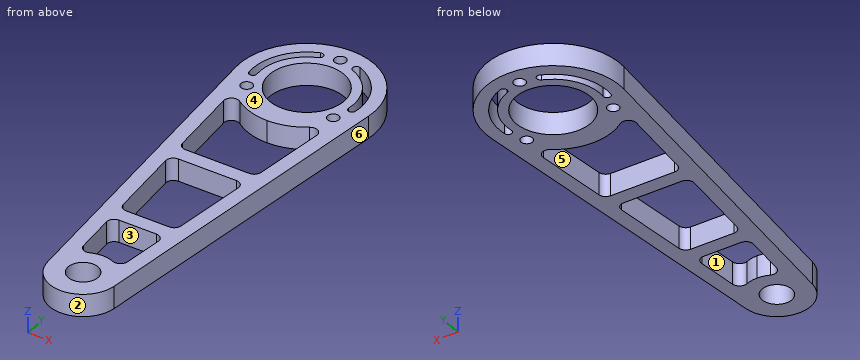
```python
from build123d import *

# Parameters (mm, degrees)
SKETCH_1_R          = 4
SKETCH_1_R_2        = 1.55
SKETCH_1_R_3        = 10
EXTRUDE_1_DEPTH     = 6
CUT_EXTRUDE_1_DEPTH = 6
EXTRUDE_2_DEPTH     = 6
FILLET_1_R          = 2
CUT_EXTRUDE_2_DEPTH = 10


with BuildPart() as part:
    # 草图1 → 凸台-拉伸1 (new body)
    with BuildSketch(Plane.XY):
        with BuildLine():
            ThreePointArc((17.909773868, -1.8), (0, 18), (-17.909773868, -1.8))
            Line((-17.909773868, -1.8), (-8.954886934, -90.9))
            ThreePointArc((-8.954886934, -90.9), (0, -99), (8.954886934, -90.9))
            Line((8.954886934, -90.9), (17.909773868, -1.8))
        make_face()
        with Locations((0, -90)):
            Circle(SKETCH_1_R, mode=Mode.SUBTRACT)
        with Locations((-11.691342951, -6.75)):
            Circle(SKETCH_1_R_2, mode=Mode.SUBTRACT)
        with Locations((11.691342951, -6.75)):
            Circle(SKETCH_1_R_2, mode=Mode.SUBTRACT)
        Circle(SKETCH_1_R_3, mode=Mode.SUBTRACT)
        with Locations((0, 13.5)):
            Circle(SKETCH_1_R_2, mode=Mode.SUBTRACT)
    extrude(amount=EXTRUDE_1_DEPTH)

    # 草图2 → 切除-拉伸1 (cut)
    with BuildSketch(Plane.XY.offset(6)):
        with BuildLine():
            ThreePointArc((13.15522745, -9.107139547), (7.425825451, -14.172406866), (0, -16))
            Line((0, -16), (0, -82))
            ThreePointArc((0, -82), (3.024106775, -82.593598835), (5.599436985, -84.286305447))
            Line((5.599436985, -84.286305447), (13.15522745, -9.107139547))
        make_face()
        with BuildLine():
            ThreePointArc((0, -16), (-7.425825451, -14.172406866), (-13.15522745, -9.107139547))
            Line((-13.15522745, -9.107139547), (-5.599436985, -84.286305447))
            ThreePointArc((-5.599436985, -84.286305447), (-3.024106775, -82.593598835), (0, -82))
            Line((0, -82), (0, -16))
        make_face()
    extrude(amount=-CUT_EXTRUDE_1_DEPTH, mode=Mode.SUBTRACT)

    # 草图3 → 凸台-拉伸2 (add)
    with BuildSketch(Plane.XY.offset(6)):
        Polygon((10.251385716, -38), (-10.251385716, -38), (-10.050378153, -40), (10.050378153, -40), align=None)
        Polygon((-10.452393279, -36), (-10.251385716, -38), (10.251385716, -38), (10.452393279, -36), align=None)
        Polygon((7.437279833, -66), (-7.437279833, -66), (-7.23627227, -68), (7.23627227, -68), align=None)
        Polygon((7.638287396, -64), (-7.638287396, -64), (-7.437279833, -66), (7.437279833, -66), align=None)
    extrude(amount=-EXTRUDE_2_DEPTH)

    # 圆角1
    fillet_1_edges = [part.edges().sort_by_distance(p)[0] for p in [
        (-13.15522745, -9.107139547, 3),
        (13.15522745, -9.107139547, 3),
        (5.599436985, -84.286305447, 3),
        (-5.599436985, -84.286305447, 3),
        (-10.050378153, -40, 3),
        (-10.452393279, -36, 3),
        (10.452393279, -36, 3),
        (10.050378153, -40, 3),
        (-7.23627227, -68, 3),
        (-7.638287396, -64, 3),
        (7.638287396, -64, 3),
        (7.23627227, -68, 3),
    ]]
    fillet(fillet_1_edges, radius=FILLET_1_R)

    # 草图4 → 切除-拉伸2 (cut)
    with BuildSketch(Plane.XY.offset(6)):
        with BuildLine():
            ThreePointArc((-4.62962963, 11.611052041), (-4.071115837, 12.910306574), (-5.37037037, 13.468820367))
            ThreePointArc((-5.37037037, 13.468820367), (-12.505593382, 7.338946393), (-14.377656014, -1.87962963))
            ThreePointArc((-14.377656014, -1.87962963), (-13.256463901, -2.741562484), (-12.394531047, -1.62037037))
            ThreePointArc((-12.394531047, -1.62037037), (-10.78068395, 6.326677925), (-4.62962963, 11.611052041))
        make_face()
        with BuildLine():
            ThreePointArc((5.37037037, 13.468820367), (12.505593382, 7.338946393), (14.377656014, -1.87962963))
            ThreePointArc((14.377656014, -1.87962963), (13.256463901, -2.741562484), (12.394531047, -1.62037037))
            ThreePointArc((12.394531047, -1.62037037), (10.78068395, 6.326677925), (4.62962963, 11.611052041))
            ThreePointArc((4.62962963, 11.611052041), (4.071115837, 12.910306574), (5.37037037, 13.468820367))
        make_face()
    extrude(amount=-CUT_EXTRUDE_2_DEPTH, mode=Mode.SUBTRACT)


solid = part.part
```
CAD build for the part. Positions are in the model's coordinates, mm. Face numbers are marked on the shaded views. A direction names the side the tool comes from. Round coordinates to 2 decimals unless told otherwise and drop trailing zeros. Loops run counter-clockwise (first coordinate to the right, second up) from the corner with the lowest first, then second, coordinate; pieces in that order, holes last. Notation, with made-up numbers: M 36.5,75.25 L 42.5,75.25 A16 ccw 42.5,83.25 Z; hole C 14.25,60.5 d11. An arc over 180 degrees is marked long. Use a Markdown table: item, result. Add a question column.
(1) Pull direction X, two halves, no side cores. Call the marked faces 1, 2, 3 and 4: +X half, -X half, draft (parallel to the pull), parting line (faces both ways), or undercut.
(2) Cut at B-B (y = -69). Give the cut face in (x, z).
(3) Cut at A-A (y = 0). Give the cut face in (x, z).
(4) Drill centre lines: line 1 (Y direction, x = -5, z = 2.7); line 2 (Y direction, x = 3, z = 3.85); line 3 (X direction, y = -53.5, z = 2). Where is each one in solid material? Low to high.
(5) Flat gauge pins, fed straight in: pin 1 (2.5 mm diameter, centred on x = 0, y = 13.5, fed in from -Z); pin 2 (1.5 mm diameter, centred on y = 3, z = 3, fed in from +X); pin 3 (1.5 mm diameter, centred on x = -6.5, z = 3.5, fed in from +Y); pin 4 (1.5 mm diameter, centred on x = -5, z = 2, fed in from -Y). Where does each tip first touch, or does it go through?
(6) Cut at D-D (y = -20). Give the cut face in (x, z), and give its area (3 significant figures).
(7) Which spindle directions (+Z, -Z, +X, -X, +Y, -Y) get a long thin tool onto all of the face, cutting with end or side? Do the marked faces 5 and 6. Say none if no direction does.
(8) Cut at C-C (z = 4.9). State how many separate pieces and enclosed holes the cut face has, and give its area (3 significant figures).
Geometry says:
| question | item | result |
|---|---|---|
| 1 | face 1 | undercut |
| 1 | face 2 | parting line |
| 1 | face 3 | undercut |
| 1 | face 4 | draft |
| 2 | outline | M -11.16,0 L -6.76,0 L -6.76,6 L -11.16,6 Z; M 6.76,0 L 11.16,0 L 11.16,6 L 6.76,6 Z |
| 3 | outline | M -18,0 L -14.5,0 L -14.5,6 L -18,6 Z; M -12.5,0 L -10,0 L -10,6 L -12.5,6 Z; M 10,0 L 12.5,0 L 12.5,6 L 10,6 Z; M 14.5,0 L 18,0 L 18,6 L 14.5,6 Z |
| 4 | line 1 | y = -97.48 to -82.5, -68 to -64, -40 to -36, -15.2 to -8.66, 8.66 to 11.46, 13.54 to 17.29 |
| 4 | line 2 | y = -98.49 to -92.65, -87.35 to -82.58, -68 to -64, -40 to -36, -15.72 to -9.54, 9.54 to 17.75 |
| 4 | line 3 | x = -12.71 to -8.69, 8.69 to 12.71 |
| 5 | pin 1 | passes through |
| 5 | pin 2 | stops at x = 17.86 |
| 5 | pin 3 | stops at y = 17.06 |
| 5 | pin 4 | stops at y = -97.93 |
| 6 | outline | M -16.08,0 L -12.06,0 L -12.06,6 L -16.08,6 Z; M 12.06,0 L 16.08,0 L 16.08,6 L 12.06,6 Z |
| 6 | area | 48.2 mm² |
| 7 | face 5 | +Z, -Z |
| 7 | face 6 | +Z, -Z, +X, -Y |
| 8 | separate pieces | 1 |
| 8 | enclosed holes | 10 |
| 8 | area | 1,510 mm² |
